Part print with two shaded views. Sizes in mm from the minimum x, y, z corner. Round coordinates to 2 decimals unless told otherwise and drop trailing zeros. Loops run counter-clockwise (first coordinate to the right, second up) from the corner with the lowest first, then second, coordinate; pieces in that order, holes last.
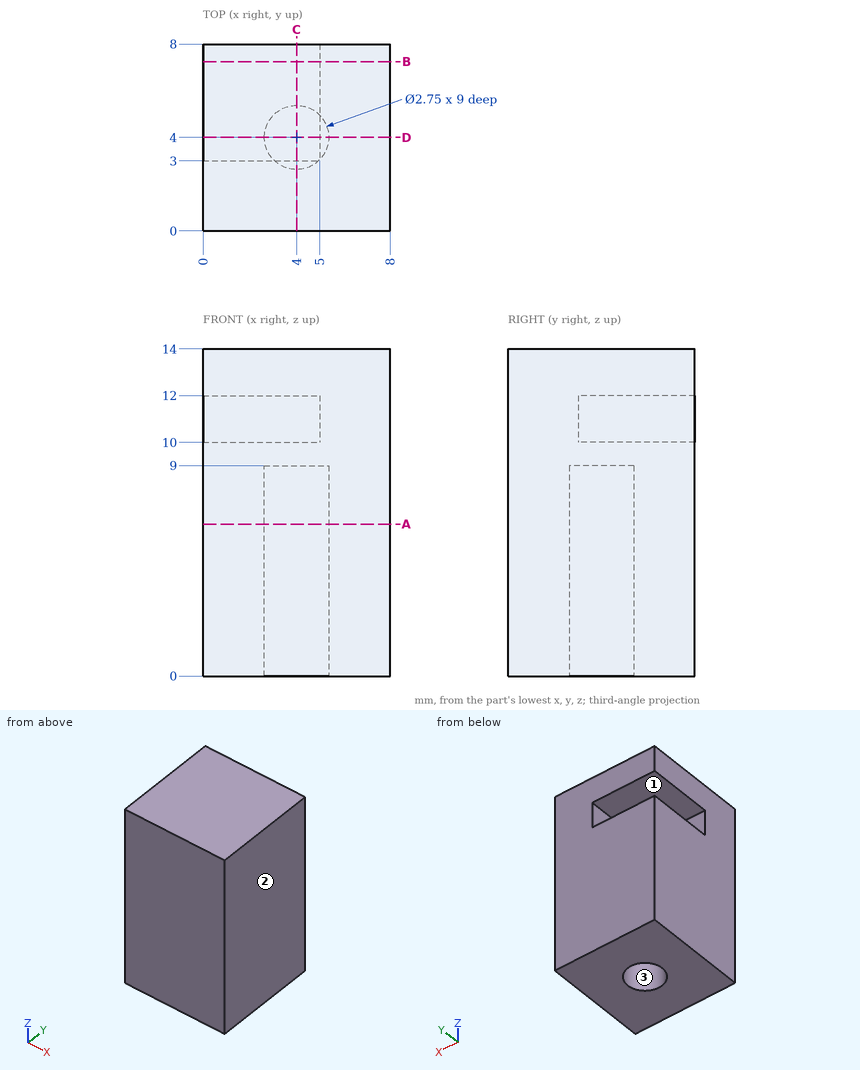
Item 1: Cut at D-D (y = 4). List the corners of the cut face in (x, z) (3 decimals), plus the area to 4 significant figures.
Verdict:
outline: (0, 0) - (2.625, 0) - (2.625, 9) - (5.375, 9) - (5.375, 0) - (8, 0) - (8, 14) - (0, 14) - (0, 12) - (5, 12) - (5, 10) - (0, 10) - close
area: 77.25 mm2
Item 2: Mould opens along X. For the marked faces 1, 2 and 3 say: released by +X, released by -X, zero draft, split by the parting line, or undercut.
Verdict:
face 1: zero draft
face 2: released by +X
face 3: undercut
Item 3: Flat gauge pins, fed straight in: P1, Ø0.6, axis at y = 4.5, z = 11, coming from the -X side; P2, Ø0.8, axis at x = 4, y = 3.5, coming from the -Z side. Where does each tip first touch, or does it go through?
Verdict:
P1: stops at x = 5
P2: stops at z = 9
Item 4: Cut at C-C (x = 4). List the corners of the cut face in (y, z) (3 decimals).
Verdict:
outline: (0, 0) - (2.625, 0) - (2.625, 9) - (5.375, 9) - (5.375, 0) - (8, 0) - (8, 10) - (3, 10) - (3, 12) - (8, 12) - (8, 14) - (0, 14) - close
Item 5: Wall check: L1, parallel to Y at x = 4, z = 5.5 (3 decimals); L2, parallel to Z at x = 2.25, y = 6.75; L3, parallel to Z at x = 3.5, y = 3.25. Give the ranges that are in metal, low to high.
Verdict:
L1: y = 0 to 2.625, 5.375 to 8
L2: z = 0 to 10, 12 to 14
L3: z = 9 to 10, 12 to 14
Item 6: Cut at B-B (y = 7.25). List the corners of the cut face in (x, z), plus the area to 3 significant figures.
Verdict:
outline: (0, 0) - (8, 0) - (8, 14) - (0, 14) - (0, 12) - (5, 12) - (5, 10) - (0, 10) - close
area: 102 mm2
Item 7: Cut at A-A (z = 6.5). List the corners of the cut face in (x, y) (3 decimals).
Verdict:
outline: (0, 0) - (8, 0) - (8, 8) - (0, 8) - close; hole circle Ø2.75 at (4, 4)
